Design review of the part built by this model. Coordinates are the model's own, in mm. Round coordinates to 2 decimals unless told otherwise and drop trailing zeros. Loops run counter-clockwise (first coordinate to the right, second up) from the corner with the lowest first, then second, coordinate; pieces in that order, holes last. Notation, with made-up numbers: (6, 81) -> (34, 81) arc R24 cw to (34, 108) -> close; hole circle Ø5 at (-21, -28). An arc over 180 degrees is marked (long way). Use a Markdown table: item, result. Add a question column.
from build123d import *

# Parameters (mm, degrees)
F0_R     = 6
F1_DEPTH = 3


# Not quite as in the source:
# - a feature names something its author has since deleted; it is built from what else it names


with BuildPart() as f1:
    # F0 (on Top) → F1 (new body)
    with BuildSketch(Plane.XY):
        with BuildLine():
            Line((-36, 29), (-76, 29))
            Line((-76, 29), (-76, -12.5))
            Line((-76, -12.5), (0, -12.5))
            ThreePointArc((0, -12.5), (12.5, 0), (0, 12.5))
            Line((0, 12.5), (-36, 29))
        make_face()
        Circle(F0_R, mode=Mode.SUBTRACT)
    extrude(amount=-F1_DEPTH)


solid = f1.part
1. Consider section B-B on z = -0.7. State the section outline as (x, y) points.
2. To check wall thickness, follow probe 1 along Y at (x, z) = (-1.5, -1.1); probe 2 along X at (y, z) = (-4.5, -0.4); probe 3 along X at (y, z) = (4, -0.1). State the ranges of each line that lie inside material, in increasing order. Write a range as from..to.
3. Consider section A-A on y = 0. State the section outline as (x, z) points.
4. Consider section C-C on x = 3. State the section outline as (y, z) points, plus the area to 3 significant figures.
5. Consider section D-D on x = -29. State the section outline as (y, z) points.
6. Insertion check: P1, Ø4, axis at x = -22.5, y = 19.5, coming from the +Z side; P2, Ø9.5, axis at x = 0, y = 0, coming from the +Z side. Each pin has a flat end and moves straight along its axis. Give the tip position at first contact, or say it passes through.
7. Mouldability with a two-part tool opening along Y and no side actions: class faces 1 (the face through (-56, 29, -1)), 2 (the face through (12.497, -0.275, -1.479)), 3 (the face through (-6, 0, -1)) as +Y half, -Y half, draft (parallel to the pull), parting line (faces both ways), or undercut.
Verdict:
| question | item | result |
|---|---|---|
| 1 | outline | (-76, -12.5) -> (0, -12.5) arc R12.5 ccw to (0, 12.5) -> (-36, 29) -> (-76, 29) -> close; hole circle Ø12 at (0, 0) |
| 2 | probe 1 | y = -12.5..-5.81, 5.81..13.19 |
| 2 | probe 2 | x = -76..-3.97, 3.97..11.66 |
| 2 | probe 3 | x = -76..-4.47, 4.47..11.84 |
| 3 | outline | (-76, -3) -> (-6, -3) -> (-6, 0) -> (-76, 0) -> close; (6, -3) -> (12.5, -3) -> (12.5, 0) -> (6, 0) -> close |
| 4 | outline | (-12.13, -3) -> (-5.2, -3) -> (-5.2, 0) -> (-12.13, 0) -> close; (5.2, -3) -> (12.13, -3) -> (12.13, 0) -> (5.2, 0) -> close |
| 4 | area | 41.6 mm² |
| 5 | outline | (-12.5, -3) -> (25.79, -3) -> (25.79, 0) -> (-12.5, 0) -> close |
| 6 | P1 | stops at z = 0 |
| 6 | P2 | passes through |
| 7 | face 1 | +Y half |
| 7 | face 2 | parting line |
| 7 | face 3 | undercut |
